Model file for the job. Use its own axes, mm. A direction names the side the tool comes from. Give positions to 0.01 mm unless a question says otherwise; leave off trailing zeros. Write each loop counter-clockwise with the first axis right and the second up, starting at its lowest first coordinate (ties: lowest second). Pieces come first, ordered by that corner, then holes. Notation, with made-up numbers: (-20, -3.75) - (23, -3.75) arc R7 cw to (23, 4.25) - close; hole circle Ø3 at (27, 16.25). An arc over 180 degrees is marked (long way). One line per item, written item: value. Start each with the question number.
(1) Cut at A-A, the plane z = 206.5. List the corners of the cut face in (x, y), and give its area (3 significant figures).
(2) Drop a flat-ended pin along its axis: P1, Ø5, axis at x = 150.5, z = -87.5, coming from the -Y side. Give the stop position or say it passes through.
(3) Cut at B-B, the plane y = -264. List the corners of the cut face in (x, z).
(4) 3-axis set-ups, long thin cutter, end or side, ignore diameter. For faces 5 (the face through (-190.5, -182, -87)), 6 (the face through (-3, -175, 381)): which of +Z, -Z, +X, -X, +Y, -Y reach the whole face in a straight line?
(5) Cut at C-C, the plane x = 32. List the corners of the cut face in (y, z).
(6) Mould opens along X. For faces 1 (the face through (-3, -182, 196.85)), 2 (the face through (-203.2, -175, -5)), 3 (the face through (-3, 0, 5)), 4 (the face through (-3, -12.7, -85)) say: pulls with the +X half, pulls with the -X half, needs draft (parallel to the pull), parting line crosses it, or undercut.
(7) Probe L1, parallel to Z at x = 181, y = -129.5; L2, parallel to X at y = -172.5, z = -39; L3, parallel to Y at x = 72, z = 159. List the from-to ranges inside material, lowest first.
from build123d import *

# Parameters (mm, degrees)
F0_W     = 406.4
F0_H     = 762
F1_DEPTH = 355.6
F2_T     = -12.7
F3_W     = 381
F3_H     = 12.7
F4_DEPTH = 342.9


with BuildPart() as f1:
    # F0 (on Front) → F1 (new body)
    with BuildSketch(Plane.XZ):
        Rectangle(F0_W, F0_H)
    extrude(amount=F1_DEPTH)

    # F2
    f2_openings = [f1.faces().sort_by_distance(p)[0] for p in [
        (0, -355.6, 0),
    ]]
    offset(amount=F2_T, openings=f2_openings)

    # F3 (on face) → F4 (join)
    with BuildSketch(Plane.XZ.offset(12.7)):
        with Locations((0, 190.5)):
            Rectangle(F3_W, F3_H)
        with Locations((0, 6.35)):
            Rectangle(F3_W, F3_H)
        with Locations((0, -177.8)):
            Rectangle(F3_W, F3_H)
    extrude(amount=F4_DEPTH)


solid = f1.part
Answers follow:
1. outline: (-203.2, -355.6) - (-190.5, -355.6) - (-190.5, -12.7) - (190.5, -12.7) - (190.5, -355.6) - (203.2, -355.6) - (203.2, 0) - (-203.2, 0) - close
1. area: 13,900 mm²
2. P1: stops at y = -12.7
3. outline: (-203.2, -381) - (203.2, -381) - (203.2, 381) - (-203.2, 381) - close; hole (-190.5, -368.3) - (190.5, -368.3) - (190.5, -184.15) - (-190.5, -184.15) - close; hole (-190.5, -171.45) - (190.5, -171.45) - (190.5, 0) - (-190.5, 0) - close; hole (-190.5, 12.7) - (190.5, 12.7) - (190.5, 184.15) - (-190.5, 184.15) - close; hole (-190.5, 196.85) - (190.5, 196.85) - (190.5, 368.3) - (-190.5, 368.3) - close
4. face 5: -Y
4. face 6: +Z, +X, -X, +Y, -Y
5. outline: (-355.6, -381) - (0, -381) - (0, 381) - (-355.6, 381) - (-355.6, 368.3) - (-12.7, 368.3) - (-12.7, 196.85) - (-355.6, 196.85) - (-355.6, 184.15) - (-12.7, 184.15) - (-12.7, 12.7) - (-355.6, 12.7) - (-355.6, 0) - (-12.7, 0) - (-12.7, -171.45) - (-355.6, -171.45) - (-355.6, -184.15) - (-12.7, -184.15) - (-12.7, -368.3) - (-355.6, -368.3) - close
6. face 1: undercut
6. face 2: pulls with the -X half
6. face 3: needs draft
6. face 4: undercut
7. L1: z = -381 to -368.3, -184.15 to -171.45, 0 to 12.7, 184.15 to 196.85, 368.3 to 381
7. L2: x = -203.2 to -190.5, 190.5 to 203.2
7. L3: y = -12.7 to 0
